Here's how the part is built. I have some questions about the finished solid (model axes, mm). A direction names the side the tool comes from. Round coordinates to 2 decimals unless told otherwise and drop trailing zeros. Order: outer loops, then holes, each group sorted by start corner. A loop starts at its lowest first (then second) coordinate and runs counter-clockwise, first axis right, second up. Notation, with made-up numbers: M -7.75,-17 L -0.75,-17 A20 ccw -0.75,22 Z; hole C -24.5,34.5 d9. An arc over 180 degrees is marked long. Use one line per item in the form item = value. Start each with the question number.
```python
from build123d import *

# Parameters (mm, degrees)
F1_DEPTH  = 58
F3_DEPTH  = 58.001
F6_DEPTH  = 42.001
F7_DEPTH  = 15
F9_DEPTH  = 42.001
F10_R     = 6
F11_DEPTH = 26


with BuildPart() as f1:
    # F0 (on Top) → F1 (new body)
    with BuildSketch(Plane.XY):
        Polygon((0, 58), (0, 0), (58, 0), (58, 16), (16, 16), (16, 42), (88, 42), (88, 16), (118, 16), (118, 58), align=None)
        Polygon((16, 16), (58, 16), (88, 16), (88, 42), (16, 42), align=None)
    extrude(amount=F1_DEPTH)

    # F2 (on face) → F3 (cut, through all)
    with BuildSketch(Plane.XZ):
        Polygon((14.689402, 58), (0, 58), (14.689402, 47.95216), align=None)
    extrude(amount=-F3_DEPTH, mode=Mode.SUBTRACT)

    # F5 (on face) → F6 (cut, through all)
    with BuildSketch(Plane.XZ.offset(-16)):
        Polygon((118, 58), (97.528502, 58), (99.474385, 12.926235), (118, 9.312449), align=None)
    extrude(amount=-F6_DEPTH, mode=Mode.SUBTRACT)

    # F4 (on face) → F7 (join, symmetric)
    with BuildSketch(Plane.XZ):
        Polygon((58, 19.875824), (14.689402, 47.95216), (0, 58), (0, 0), (58, 0), align=None)
    extrude(amount=F7_DEPTH, both=True)

    # F8 (on face) → F9 (cut, through all)
    with BuildSketch(Plane.XZ.offset(-16)):
        Polygon((97.528502, 58), (58, 58), (58, 20.431791), (99.474385, 12.926235), align=None)
    extrude(amount=-F9_DEPTH, mode=Mode.SUBTRACT)

    # F10 (on face) → F11 (cut)
    with BuildSketch(Plane.XZ):
        with Locations((42, 44.894345)):
            Circle(F10_R)
    extrude(amount=-F11_DEPTH, mode=Mode.SUBTRACT)


solid = f1.part
```
1) If we mould it in two halves opening along Z, with no side actions, what happens to faces 1 (the flat face through (45, 30, 0)), 2 (the cylindrical face through (36, 13, 45)), 3 (the flat face through (14.689, 29, 53)), 4 (the flat face through (42, 26, 45))? For each: +Z half, -Z half, draft (parallel to the pull), parting line (faces both ways), or undercut.
2) On a 3-axis mill with a long thin cutter (end or side, diameter ignored), from which of +Z, -Z, +X, -X, +Y, -Y can I reach the whole of each face in a straight line? I mean faces 5 (the flat face through (58, 21, 35)), 6 (the flat face through (78.45, 36.71, 16.73)), 7 (the flat face through (7.24, 20.99, 53.05)), 8 (the flat face through (81, 16, 8)). Say none if no direction works.
3) If we section it at D-D on z = 32.5: Write out the boundary of the cut face in (x, y).
4) If I drill on line 1 (Z direction, x = 42, y = 16); line 2 (X direction, y = 2, z = 29.5); line 3 (X direction, y = 53.5, z = 49), over which ranges is the centre line in solid material (lowest first)?
5) If we section it at A-A on y = 31.5: Write out the boundary of the cut face in (x, z), then the cut area to 3 significant figures.
6) If we section it at C-C on y = 2: Write out the boundary of the cut face in (x, z), then the cut area to 3 significant figures.
7) If we section it at B-B on x = 42: Write out the boundary of the cut face in (y, z), then the cut area to 3 significant figures.
8) Will these pins go through, and if not, where does the flat tip stop? pin 1 Ø3 at (x, y) = (97.5, 17) entering from +Z (3 decimals); pin 2 Ø8 at (y, z) = (27, 10.5) entering from +X; pin 3 Ø13 at (x, z) = (40.5, 43) entering from -Y; pin 4 Ø6 at (x, z) = (88.5, 10) entering from -Y.
Completed:
q1.face_1 = -Z half
q1.face_2 = undercut
q1.face_3 = draft
q1.face_4 = undercut
q2.face_5 = +Z, +X, -Y
q2.face_6 = +Z, +X, +Y, -Y
q2.face_7 = +Z, +Y, -Y
q2.face_8 = +Z, -Z, +X, -Y
q3.outline = M 0,-15 L 38.53,-15 L 38.53,0 L 58,0 L 58,58 L 0,58 Z
q4.line_1 = 0 to 38.89, 50.89 to 58
q4.line_2 = 0 to 58
q4.line_3 = 0 to 13.16, 14.69 to 58
q5.outline = M 0,0 L 118,0 L 118,9.31 L 99.47,12.93 L 58,20.43 L 58,58 L 14.69,58 L 14.69,47.95 L 0,58 Z
q5.area = 4,190 mm²
q6.outline = M 0,0 L 58,0 L 58,58 L 14.69,58 L 14.69,47.95 L 0,58 Z; hole C 42,44.89 d12
q6.area = 3,180 mm²
q7.outline = M -15,0 L 58,0 L 58,58 L 0,58 L 0,50.89 L 26,50.89 L 26,38.89 L 0,38.89 L 0,30.25 L -15,30.25 Z
q7.area = 3,510 mm²
q8.pin_1 = 13.555
q8.pin_2 = 118
q8.pin_3 = 0
q8.pin_4 = 16
